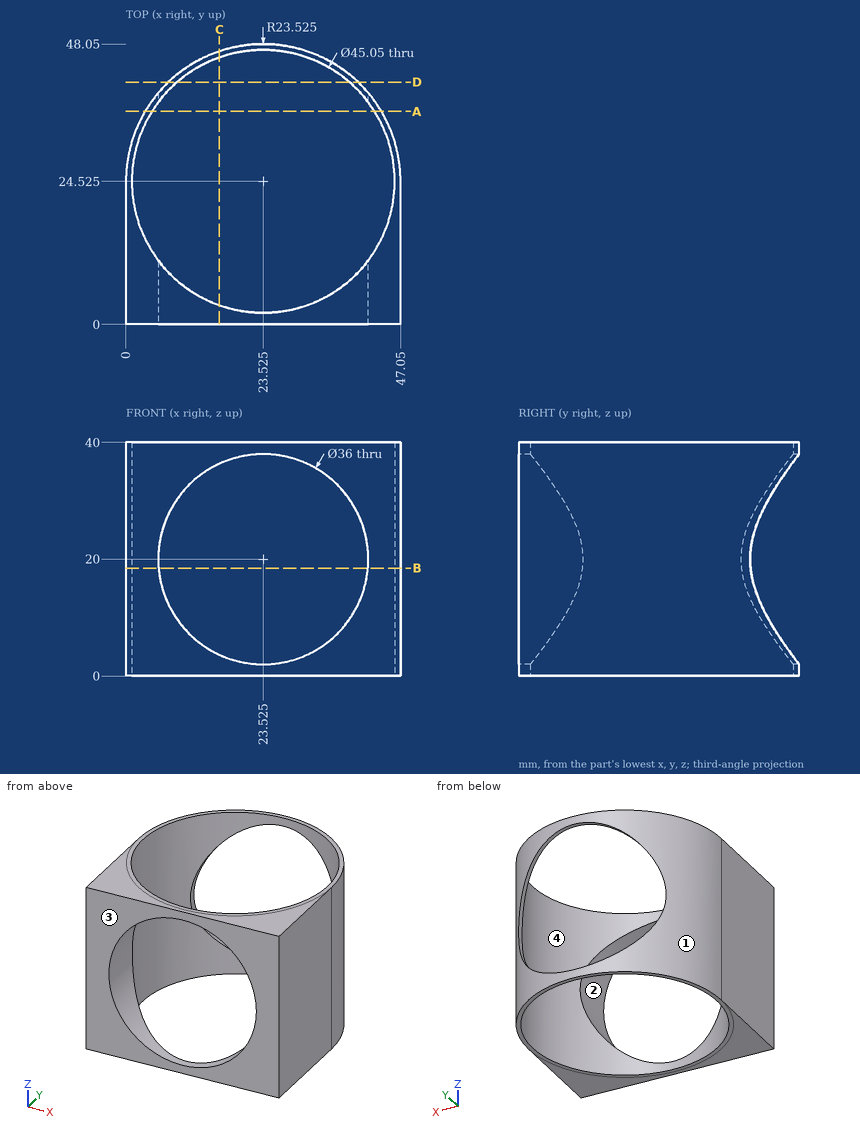
For this review, use the dimensioned drawing (mm, ordinates from the lowest corner) and the shaded views. Give positions to 0.01 mm unless a question says otherwise; leave off trailing zeros. Write each loop counter-clockwise with the first axis right and the second up, starting at its lowest first coordinate (ties: lowest second). Pieces come first, ordered by that corner, then holes. Notation, with made-up numbers: M 67,-6 L 75,-6 A25 ccw 75,14 Z; hole C 21.5,40.25 d6. An arc over 180 degrees is marked long. Answer as a JSON object with one key per item and string values. Group by question number.
Item 1: Consider section D-D on y = 41.5. Write out the cut boundary in (x, z) (3 decimals).
Item 2: Consider section A-A on y = 36.5. Write out the cut boundary in (x, z), plus the area to 3 significant figures.
Item 3: Consider section C-C on x = 16. Write out the cut boundary in (y, z).
Item 4: For probe 1 along X at (y, z) = (31, 36); probe 2 along Y at (x, z) = (4.5, 10); probe 3 along X at (y, z) = (3, 18), list the stretches that pass through material, from the lowest coordinate up. Write a range as [from, to].
Item 5: For pin 1 Ø4 at (y, z) = (29, 22) entering from +X; pin 2 Ø10 at (x, y) = (36, 35) entering from +Z, all flat-tipped, find the tip position at first contact; note any pin that passes through.
Item 6: Draft analysis for pull direction X (two halves, no side actions). For the marked faces 1, 2, 3 and 4, state which applies: +X half, -X half, draft (parallel to the pull), parting line (faces both ways), or undercut.
Item 7: Consider section B-B on z = 18.5. Write out the cut boundary in (x, y) (3 decimals), plus the area to 3 significant figures.
Check result:
{
 "1": {"outline": "M 7.238,0 L 8.719,0 L 8.719,9.764 A18 cw 7.238,12.337 Z; M 7.238,27.663 A18 cw 8.719,30.236 L 8.719,40 L 7.238,40 Z; M 38.331,0 L 39.812,0 L 39.812,12.337 A18 cw 38.331,9.764 Z; M 38.331,30.236 A18 cw 39.812,27.663 L 39.812,40 L 38.331,40 Z"},
 "2": {"outline": "M 3.28,0 L 4.45,0 L 4.45,40 L 3.28,40 Z; M 42.6,0 L 43.77,0 L 43.77,40 L 42.6,40 Z", "area": "93.7 mm^2"},
 "3": {"outline": "M 0,0 L 3.29,0 L 3.29,3.65 L 0,3.65 Z; M 0,36.35 L 3.29,36.35 L 3.29,40 L 0,40 Z; M 45.76,0 L 46.81,0 L 46.81,3.65 L 45.76,3.65 Z; M 45.76,36.35 L 46.81,36.35 L 46.81,40 L 45.76,40 Z"},
 "4": {"probe 1": "x = [0.91, 1.95], [45.1, 46.14]", "probe 2": "y = [0, 12.47], [36.58, 38.36]", "probe 3": "x = [0, 5.64], [41.41, 47.05]"},
 "5": {"pin 1": "stops at x = 46.92", "pin 2": "passes through"},
 "6": {"face 1": "parting line", "face 2": "undercut", "face 3": "draft", "face 4": "undercut"},
 "7": {"outline": "M 0,0 L 5.588,0 L 5.588,10.901 A22.525 cw 5.588,38.149 L 5.588,39.746 A23.525 ccw 0,24.525 Z; M 41.462,0 L 47.05,0 L 47.05,24.525 A23.525 ccw 41.462,39.746 L 41.462,38.149 A22.525 cw 41.462,10.901 Z", "area": "220 mm^2"}
}
